Can you work these out from the model? Positions are in its coordinate system, mm. A direction names the side the tool comes from. Round coordinates to 2 decimals unless told otherwise and drop trailing zeros. Write each loop counter-clockwise with the first axis right and the second up, starting at its lowest first coordinate (ties: lowest second). Pieces come first, ordered by that corner, then holes. Notation, with made-up numbers: M -16,41.5 L -8,41.5 A14 cw -8,58.5 Z; hole C 46.5,45.25 d4. An arc over 180 degrees is marked long. Answer as a JSON object with one key per item and string values. Group by question number.
1) Please list where these lines run through material, in increasing order: L1, parallel to Z at x = 8.25, y = -10.25 (1 decimal); L2, parallel to Y at x = 12, z = 40.5; L3, parallel to X at y = -28, z = 57. Write a range as [from, to].
2) I'm going to push a flat-ended pin straight in: pin 1 Ø7 at (x, z) = (8.25, 34.925) entering from -Y. Where does the tip first touch, or does it pass through?
3) Suppose I cut it at C-C, the plane z = 37. Write out the boundary of the cut face in (x, y).
4) Suppose I cut it at D-D, the plane x = 27.3. Write out the boundary of the cut face in (y, z).
5) If we mould it in two halves opening along X, with no side actions, what happens to faces 3 (the cylindrical face through (8.64, -12.67, 31.95)), 4 (the flat face through (20, -25, 35)), 5 (the flat face through (0, -12, 35))? For each: +X half, -X half, draft (parallel to the pull), parting line (faces both ways), or undercut.
6) On a 3-axis mill with a long thin cutter (end or side, diameter ignored), from which of +Z, -Z, +X, -X, +Y, -Y can I reach the whole of each face in a straight line? I mean faces 1 (the cylindrical face through (30.995, -39.79, 55.618)), 2 (the flat face through (20, 0, 35)). Say none if no direction works.
7) Suppose I cut it at B-B, the plane z = 57.15. Write out the boundary of the cut face in (x, y).
8) Suppose I cut it at A-A, the plane x = 8.25. Write out the boundary of the cut face in (y, z) (1 decimal).
from build123d import *

# Parameters (mm, degrees)
F0_W     = 40
F0_H     = 70
F1_DEPTH = 25
F2_R     = 4
F3_DEPTH = 30
F6_D     = 6


# Not quite as in the source:
# - the program builds the solid bodies; features that only make, move or delete a surface that nothing else refers to are left out


with BuildPart() as f1:
    # F0 (on Front) → F1 (new body)
    with BuildSketch(Plane.XZ):
        with Locations((20, 35)):
            Rectangle(F0_W, F0_H)
    extrude(amount=F1_DEPTH)

    # F2 (on face) → F3 (join)
    with BuildSketch(Plane.XZ.offset(25)):
        with Locations((27.3, 57.15)):
            Circle(F2_R)
    extrude(amount=F3_DEPTH)

    # F6 (through all)
    with Locations(Plane(origin=(0, 0, 0), x_dir=(1, 0, 0), z_dir=(0, 1, 0))):
        with Locations((8.25, -52.3875), (8.25, -34.925)):
            Hole(F6_D / 2)


solid = f1.part
Results:
{
 "1": {"L1": "[0, 31.9], [37.9, 49.4], [55.4, 70]", "L2": "[-25, 0]", "L3": "[23.3, 31.3]"},
 "2": {"pin 1": "y = -25"},
 "3": {"outline": "M 0,-25 L 6.08,-25 L 6.08,0 L 0,0 Z; M 10.42,-25 L 40,-25 L 40,0 L 10.42,0 Z"},
 "4": {"outline": "M -55,53.15 L -25,53.15 L -25,0 L 0,0 L 0,70 L -25,70 L -25,61.15 L -55,61.15 Z"},
 "5": {"face 3": "undercut", "face 4": "draft", "face 5": "-X half"},
 "6": {"face 1": "-Y", "face 2": "+Z, -Z, +X, -X, +Y"},
 "7": {"outline": "M 0,-25 L 23.3,-25 L 23.3,-55 L 31.3,-55 L 31.3,-25 L 40,-25 L 40,0 L 0,0 Z"},
 "8": {"outline": "M -25,0 L 0,0 L 0,31.9 L -25,31.9 Z; M -25,37.9 L 0,37.9 L 0,49.4 L -25,49.4 Z; M -25,55.4 L 0,55.4 L 0,70 L -25,70 Z"}
}
